Answer from the drawing. Dimensions are ordinates in mm from the lowest x, y and z of the part. Coordinates: 2 decimals unless noted, no trailing zeros. Order: outer loops, then holes, each group sorted by start corner. A loop starts at its lowest first (then second) coordinate and runs counter-clockwise, first axis right, second up. Notation, with made-up numbers: (62.5, -10) -> (92.5, -10) arc R13 cw to (92.5, -2) -> close; hole circle Ø7 at (1, -0.5). An arc over 180 degrees is marked (long way). Answer as a JSON object with one key per item and string values. Group by question number.
1) Determine the mould class of the marked faces 1, 2, 3 and 4 for opening direction X: released by +X, released by -X, zero draft, split by the parting line, or undercut.
2) Section A-A on y = 45 is taken. Determine the outline of the cut face in (x, z).
3) Given pin 1 (12 mm diameter, centred on x = 23, y = 38, fed in from +Z); pin 2 (3 mm diameter, centred on x = 35, z = 25, fed in from -Y); pin 3 (2.5 mm diameter, centred on x = 5, z = 25, fed in from -Y); pin 4 (5.5 mm diameter, centred on y = 55, z = 15, fed in from +X), each flat-ended and moving along its own axis, determine where each tip first touches the part or whether it passes through.
4) Section B-B on x = 22 is taken. Count the separate pieces of the cut face and the enclosed holes in it.
5) Section D-D on y = 9 is taken. Determine the outline of the cut face in (x, z).
6) Section C-C on z = 15 is taken. Determine the outline of the cut face in (x, y).
7) Consider L1, parallel to Z at x = 5, y = 4.5; L2, parallel to X at y = 12.25, z = 25; L3, parallel to Y at x = 24, z = 6.75. Determine where each line is inside the solid, lowest interval first.
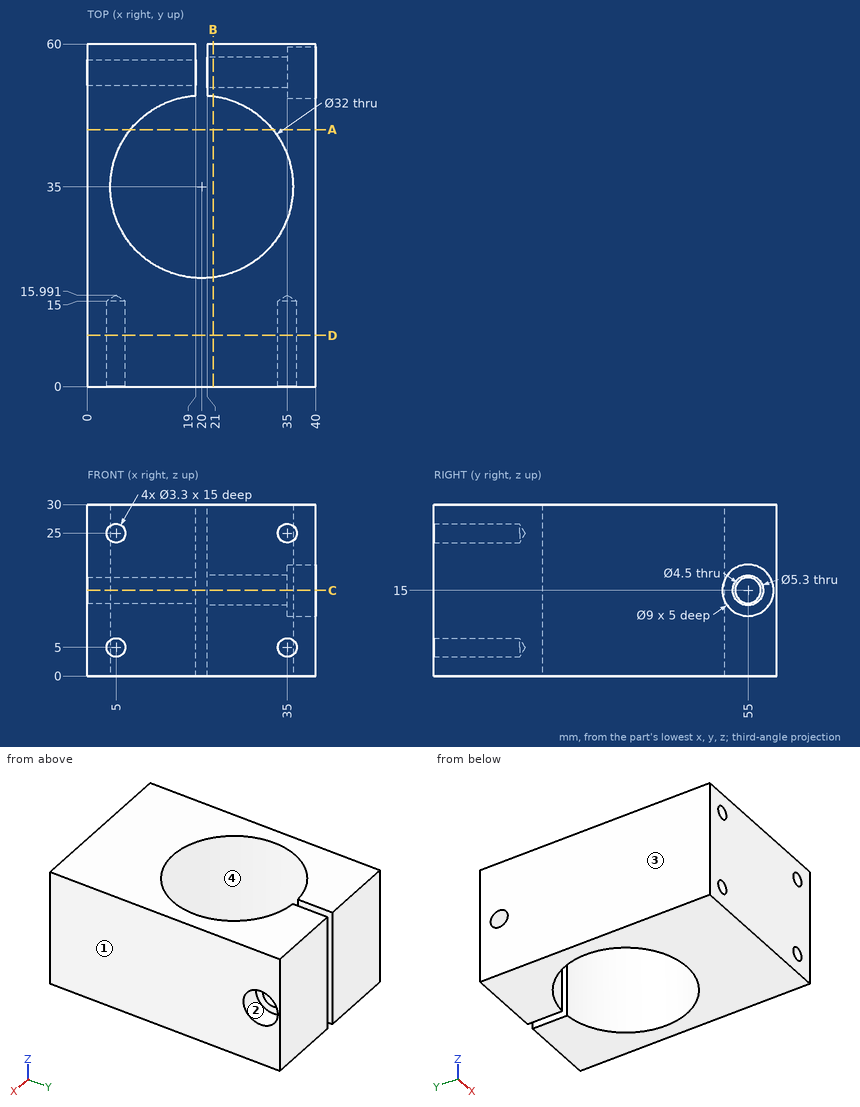
Worked answers:
{
 "1": {"face 1": "released by +X", "face 2": "zero draft", "face 3": "released by -X", "face 4": "undercut"},
 "2": {"outline": "(0, 0) -> (7.51, 0) -> (7.51, 30) -> (0, 30) -> close; (32.49, 0) -> (40, 0) -> (40, 30) -> (32.49, 30) -> close"},
 "3": {"pin 1": "passes through", "pin 2": "stops at y = 15.09", "pin 3": "stops at y = 15.24", "pin 4": "stops at x = 35"},
 "4": {"separate pieces": "2", "enclosed holes": "1"},
 "5": {"outline": "(0, 0) -> (40, 0) -> (40, 30) -> (0, 30) -> close; hole circle Ø3.3 at (5, 5); hole circle Ø3.3 at (5, 25); hole circle Ø3.3 at (35, 5); hole circle Ø3.3 at (35, 25)"},
 "6": {"outline": "(0, 0) -> (40, 0) -> (40, 50.5) -> (35, 50.5) -> (35, 52.35) -> (21, 52.35) -> (21, 50.97) arc R16 cw (long way) to (19, 50.97) -> (19, 52.75) -> (0, 52.75) -> close; (0, 57.25) -> (19, 57.25) -> (19, 60) -> (0, 60) -> close; (21, 57.65) -> (35, 57.65) -> (35, 59.5) -> (40, 59.5) -> (40, 60) -> (21, 60) -> close"},
 "7": {"L1": "z = 0 to 3.35, 6.65 to 23.35, 26.65 to 30", "L2": "x = 0 to 3.35, 6.65 to 33.35, 36.65 to 40", "L3": "y = 0 to 19.51, 50.49 to 60"}
}
